Read the model definition and answer for the solid it produces. Units are mm, in the model's axes. A direction names the side the tool comes from. Give positions to 0.01 mm unless a question says otherwise; leave off trailing zeros. Loops run counter-clockwise (first coordinate to the right, second up) from the corner with the lowest first, then second, coordinate; pieces in that order, holes last. Notation, with made-up numbers: (68.5, -18) - (88.5, -18) arc R15 cw to (88.5, 1) - close; hole circle Ø4 at (-15.5, 80.25). An arc over 180 degrees is marked (long way). Put each result on its own line as item: value. Start each with the question number.
1. A cutting plane is placed at C-C, the plane x = -6. Determine the outline of the cut face in (y, z).
2. Consider L1, parallel to X at y = -19.5, z = 0; L2, parallel to X at y = 1.75, z = 0; L3, parallel to X at y = -19.75, z = -4.25. Determine where each line is inside the solid, lowest interval first. Write a range as from..to.
3. A cutting plane is placed at A-A, the plane z = 6.5. Determine the outline of the cut face in (x, y), plus the area to 3 significant figures.
4. For faces 5 (the cylindrical face through (-5.78, 6.99, -7.54)), 6 (the cylindrical face through (-2.703, -20.014, 8.584)), 7 (the cylindrical face through (9.26, -18.51, 1.22)), 8 (the cylindrical face through (-5.37, 6.49, -1.19)), determine the directions among +Z, -Z, +X, -X, +Y, -Y from which every point of the face is accessible in a straight line to the end or side of a thin tool.
5. For a pull along Y with two mould halves and no side action, classify faces 1 (the flat face through (-7, 8, -6)), 2 (the flat face through (7, -21, -6)), 3 (the cylindrical face through (9.26, 5.49, 1.22)), 4 (the cylindrical face through (5.78, -20.01, -7.54)) as released by +Y, released by -Y, zero draft, split by the parting line, or undercut.
6. Given pin 1 Ø3 at (y, z) = (-12.5, 6) entering from -X; pin 2 Ø5.5 at (x, z) = (-1, -1.5) entering from +Y; pin 3 Ø2 at (y, z) = (-16, -7.5) entering from +X; pin 4 Ø4 at (x, z) = (-6, 1.5) entering from -Y, each flat-ended and moving along its own axis, determine where each tip first touches the part or whether it passes through.
7. A cutting plane is placed at B-B, the plane y = -8.5. Determine the outline of the cut face in (x, z), plus the area to 3 significant figures.
```python
from build123d import *

# Parameters (mm, degrees)
SKETCH1_R            = 5.484091061
SKETCH1_R_2          = 5
BOSS_EXTRUDE1_DEPTH  = 6
SKETCH2_R            = 9.5
SKETCH2_R_2          = 9
BOSS_EXTRUDE2_DEPTH  = 2
SKETCH3_R            = 9.341445955
BOSS_EXTRUDE5_DEPTH  = 6
SKETCH4_R            = 9.341445955
CUT_EXTRUDE1_DEPTH   = 5
BOSS_EXTRUDE7_START  = 23
SKETCH5_R            = 9.5
BOSS_EXTRUDE7_DEPTH  = 23
BOSS_EXTRUDE8_START  = 1
SKETCH7_R            = 9.341445955
BOSS_EXTRUDE8_DEPTH  = 1
BOSS_EXTRUDE9_START  = 2
SKETCH8_R            = 9.5
BOSS_EXTRUDE9_DEPTH  = 2
SKETCH9_R            = 5
CUT_EXTRUDE2_DEPTH   = 29
SKETCH10_R           = 9
SKETCH10_R_2         = 5
CUT_EXTRUDE3_DEPTH   = 2
SKETCH11_R           = 5.5
SKETCH11_R_2         = 5
BOSS_EXTRUDE10_DEPTH = 1
BOSS_EXTRUDE11_START = 1
SKETCH12_R           = 5.5
SKETCH12_R_2         = 5
BOSS_EXTRUDE11_DEPTH = 1


with BuildPart() as part:
    # Sketch1 → Boss-Extrude1 (new body)
    with BuildSketch(Plane(origin=(0, 0, 0), x_dir=(1, 0, 0), z_dir=(0, 1, 0))):
        with Locations(Location((0, 0, 0), (0, 0, 270))):
            Circle(SKETCH1_R)
        with Locations(Location((0, 0, 0), (0, 0, 270))):
            Circle(SKETCH1_R_2, mode=Mode.SUBTRACT)
    extrude(amount=BOSS_EXTRUDE1_DEPTH)



with BuildPart() as body_2:
    # Sketch2 → Boss-Extrude2 (new body)
    with BuildSketch(Plane(origin=(0, 6, 0), x_dir=(1, 0, 0), z_dir=(0, 1, 0))):
        with Locations(Location((0, 0, 0), (0, 0, 270))):
            Circle(SKETCH2_R)
        with Locations(Location((0, 0, 0), (0, 0, 270))):
            Circle(SKETCH2_R_2, mode=Mode.SUBTRACT)
    extrude(amount=BOSS_EXTRUDE2_DEPTH)


with BuildPart() as part_1:
    add(part.part)

    add(body_2.part)  # Boss-Extrude5 merges body 2
    # Sketch3 → Boss-Extrude5 (add)
    with BuildSketch(Plane.XZ):
        with Locations(Location((0, 0, 0), (0, 0, 270))):
            Circle(SKETCH3_R)
    extrude(amount=-BOSS_EXTRUDE5_DEPTH)

    # Sketch4 → Cut-Extrude1 (cut)
    with BuildSketch(Plane.XZ):
        with Locations(Location((0, 0, 0), (0, 0, 270))):
            Circle(SKETCH4_R)
    extrude(amount=-CUT_EXTRUDE1_DEPTH, mode=Mode.SUBTRACT)

    # Sketch5 → Boss-Extrude7 (add)
    with BuildSketch(Plane.XZ.offset(-5).offset(BOSS_EXTRUDE7_START)):
        with Locations(Location((0, 0, 0), (0, 0, 90))):
            Circle(SKETCH5_R)
    extrude(amount=-BOSS_EXTRUDE7_DEPTH)

    # Sketch7 → Boss-Extrude8 (add)
    with BuildSketch(Plane.XZ.offset(18).offset(BOSS_EXTRUDE8_START)):
        with Locations(Location((0, 0, 0), (0, 0, 270))):
            Circle(SKETCH7_R)
    extrude(amount=-BOSS_EXTRUDE8_DEPTH)

    # Sketch8 → Boss-Extrude9 (add)
    with BuildSketch(Plane.XZ.offset(19).offset(BOSS_EXTRUDE9_START)):
        with Locations(Location((0, 0, 0), (0, 0, 90))):
            Circle(SKETCH8_R)
    extrude(amount=-BOSS_EXTRUDE9_DEPTH)

    # Sketch9 → Cut-Extrude2 (cut)
    with BuildSketch(Plane.XZ.offset(21)):
        with Locations(Location((0, 0, 0), (0, 0, 270))):
            Circle(SKETCH9_R)
    extrude(amount=-CUT_EXTRUDE2_DEPTH, mode=Mode.SUBTRACT)

    # Sketch10 → Cut-Extrude3 (cut)
    with BuildSketch(Plane.XZ.offset(21)):
        with Locations(Location((0, 0, 0), (0, 0, 90))):
            Circle(SKETCH10_R)
        with Locations(Location((0, 0, 0), (0, 0, 270))):
            Circle(SKETCH10_R_2, mode=Mode.SUBTRACT)
    extrude(amount=-CUT_EXTRUDE3_DEPTH, mode=Mode.SUBTRACT)

    # Sketch11 → Boss-Extrude10 (add)
    with BuildSketch(Plane(origin=(0, 6, 0), x_dir=(1, 0, 0), z_dir=(0, 1, 0))):
        with Locations(Location((0, 0, 0), (0, 0, 270))):
            Circle(SKETCH11_R)
        with Locations(Location((0, 0, 0), (0, 0, 90))):
            Circle(SKETCH11_R_2, mode=Mode.SUBTRACT)
    extrude(amount=BOSS_EXTRUDE10_DEPTH)

    # Sketch12 → Boss-Extrude11 (add)
    with BuildSketch(Plane.XZ.offset(19).offset(BOSS_EXTRUDE11_START)):
        with Locations(Location((0, 0, 0), (0, 0, 90))):
            Circle(SKETCH12_R)
        with Locations(Location((0, 0, 0), (0, 0, 270))):
            Circle(SKETCH12_R_2, mode=Mode.SUBTRACT)
    extrude(amount=-BOSS_EXTRUDE11_DEPTH)


solid = part_1.part
```
Return value:
1. outline: (-21, -7.37) - (-19, -7.37) - (-19, -7.16) - (-18, -7.16) - (-18, -7.37) - (5, -7.37) - (5, -7.16) - (6, -7.16) - (6, -7.37) - (8, -7.37) - (8, -6.71) - (6, -6.71) - (6, 6.71) - (8, 6.71) - (8, 7.37) - (6, 7.37) - (6, 7.16) - (5, 7.16) - (5, 7.37) - (-18, 7.37) - (-18, 7.16) - (-19, 7.16) - (-19, 7.37) - (-21, 7.37) - (-21, 6.71) - (-19, 6.71) - (-19, -6.71) - (-21, -6.71) - close
2. L1: x = -9.5..-9, -5.5..-5, 5..5.5, 9..9.5
2. L2: x = -9.5..-5, 5..9.5
2. L3: x = -8.5..-7.93, -3.49..-2.63, 2.63..3.49, 7.93..8.5
3. outline: (-6.93, -21) - (-6.22, -21) - (-6.22, -19) - (6.22, -19) - (6.22, -21) - (6.93, -21) - (6.93, -19) - (6.71, -19) - (6.71, -18) - (6.93, -18) - (6.93, 5) - (6.71, 5) - (6.71, 6) - (6.93, 6) - (6.93, 8) - (6.22, 8) - (6.22, 6) - (-6.22, 6) - (-6.22, 8) - (-6.93, 8) - (-6.93, 6) - (-6.71, 6) - (-6.71, 5) - (-6.93, 5) - (-6.93, -18) - (-6.71, -18) - (-6.71, -19) - (-6.93, -19) - close
3. area: 351 mm2
4. face 5: +Y, -Y
4. face 6: -Y
4. face 7: none
4. face 8: +Y
5. face 1: released by +Y
5. face 2: released by -Y
5. face 3: undercut
5. face 4: zero draft
6. pin 1: stops at x = -8.37
6. pin 2: passes through
6. pin 3: stops at x = 6.93
6. pin 4: stops at y = -20
7. outline: circle Ø19 at (0, 0); hole circle Ø10 at (0, 0)
7. area: 205 mm2
